from build123d import *

# Parameters (mm, degrees)
F2_SIZE       = 2.54
F3_W          = 50.8
F3_H          = 7.62
F4_DEPTH      = 42.672
F6_R          = 3.9624
F7_DEPTH      = 38.608
F7_DEPTH_BACK = 9.398
F8_COUNT      = 8


with BuildPart() as f1:
    # F0 (on Top) → F1 (revolve)
    with BuildSketch(Plane.XY):
        Polygon((0, 25.4), (0, 44.45), (-15.748, 44.45), (-15.748, 12.7), (38.1, 12.7), (38.1, 19.05), (23.241, 19.05), (23.241, 25.4), align=None)
    revolve(axis=Axis((76.2, 0, 0), (1, 0, 0)))

    # F2
    f2_edges = [f1.edges().sort_by_distance(p)[0] for p in [
        (38.1, -19.05, 0),
        (23.241, -25.4, 0),
        (-15.748, -44.45, 0),
    ]]
    chamfer(f2_edges, length=F2_SIZE)


with BuildPart() as f4:
    # F3 (on Front) → F4 (new body, symmetric)
    with BuildSketch(Plane.XZ):
        with Locations((53.34, 0)):
            Rectangle(F3_W, F3_H)
    extrude(amount=F4_DEPTH, both=True)


with BuildPart() as f1_1:
    add(f1.part)

    # F5: cut F4
    add(f4.part, mode=Mode.SUBTRACT)


with BuildPart() as f7:
    # F6 (on face) → F7 (new body, two sides)
    with BuildSketch(Plane.YZ) as f7_sk:
        with Locations((0, -38.735)):
            Circle(F6_R)
    extrude(amount=-F7_DEPTH)
    extrude(f7_sk.sketch, amount=F7_DEPTH_BACK)


with BuildPart() as f8_1:
    # F8: instance of F7
    add(f7.part.rotate(Axis((-15.748, 0, 0), (1, 0, 0)), 1 * 360 / F8_COUNT))


with BuildPart() as f8_2:
    # F8: instance of F7
    add(f7.part.rotate(Axis((-15.748, 0, 0), (1, 0, 0)), 2 * 360 / F8_COUNT))


with BuildPart() as f8_3:
    # F8: instance of F7
    add(f7.part.rotate(Axis((-15.748, 0, 0), (1, 0, 0)), 3 * 360 / F8_COUNT))


with BuildPart() as f8_4:
    # F8: instance of F7
    add(f7.part.rotate(Axis((-15.748, 0, 0), (1, 0, 0)), 4 * 360 / F8_COUNT))


with BuildPart() as f8_5:
    # F8: instance of F7
    add(f7.part.rotate(Axis((-15.748, 0, 0), (1, 0, 0)), 5 * 360 / F8_COUNT))


with BuildPart() as f8_6:
    # F8: instance of F7
    add(f7.part.rotate(Axis((-15.748, 0, 0), (1, 0, 0)), 6 * 360 / F8_COUNT))


with BuildPart() as f8_7:
    # F8: instance of F7
    add(f7.part.rotate(Axis((-15.748, 0, 0), (1, 0, 0)), 7 * 360 / F8_COUNT))


with BuildPart() as f1_2:
    add(f1_1.part)

    # F9: cut F8_5, F7, F8_1, F8_4, F8_7, F8_6, F8_2, F8_3
    add(f8_5.part, mode=Mode.SUBTRACT)
    add(f7.part, mode=Mode.SUBTRACT)
    add(f8_1.part, mode=Mode.SUBTRACT)
    add(f8_4.part, mode=Mode.SUBTRACT)
    add(f8_7.part, mode=Mode.SUBTRACT)
    add(f8_6.part, mode=Mode.SUBTRACT)
    add(f8_2.part, mode=Mode.SUBTRACT)
    add(f8_3.part, mode=Mode.SUBTRACT)


solid = f1_2.part
Work out the finished part from the listing and answer in its coordinate system (mm). A direction names the side the tool comes from. Round coordinates to 2 decimals unless told otherwise and drop trailing zeros. Write each loop counter-clockwise with the first axis right and the second up, starting at its lowest first coordinate (ties: lowest second). Pieces come first, ordered by that corner, then holes. Notation, with made-up numbers: (13.25, -39) -> (70.25, -39) arc R26 cw to (70.25, -25) -> close; hole circle Ø2 at (62.5, 18.25). An arc over 180 degrees is marked (long way). Answer as CSV lines item,"result". Start each with the question number.
(1) A tool of negligible diameter and unlimited length cuts with its end or side. For faces 4 (the cylindrical face through (29.31, 18.17, 5.72)), 5 (the flat face through (33, -15, 3.81)), 6 (the cylindrical face through (-7.8, -30.1, -24.5)), from which of +Z, -Z, +X, -X, +Y, -Y can it reach the whole face along a straight path? Write none if from no direction.
(2) Each of these flat-tipped pins is pushed along its axis until it touches: pin 1 (10.5 mm diameter, centred on y = -27.39, z = -27.39, fed in from -X); pin 2 (12 mm diameter, centred on x = 19, y = 8.5, fed in from +Z); pin 3 (10 mm diameter, centred on x = 9, z = -16.5, fed in from -Y); pin 4 (10 mm diameter, centred on x = 19, z = -26, fed in from -Y). Where does it stop, or does it pass through?
(3) The part is cut by section A-A, the plane z = 0. Give the vertices of the cut face in (x, y).
(4) The part is cut by section C-C, the plane y = 0. Give the vertices of the cut face in (x, z).
(5) Find the intervals of material crossed by probe 1 along Z at (x, y) = (-6, 0); probe 2 along Z at (x, y) = (-1.5, -1); probe 3 along Z at (x, y) = (-8.5, 26.5), in increasing order.
(6) The part is cut by section B-B, the plane x = -7.5. Give the number of separate pieces and of enclosed holes in the cut face, then the cut area to 3 significant figures.
(7) The mould has two halves that part along Y. Classify faces 1 (the cylindrical face through (-6.696, 42.397, 13.352)), 2 (the flat face through (27.94, 16, 0)), 3 (the cylindrical face through (-7.8, 24.5, -30.1)): +Y half, -Y half, draft (parallel to the pull), parting line (faces both ways), or undercut.
Output values:
1,face 4,"+X"
1,face 5,"+X, +Y, -Y"
1,face 6,"+X, -X"
2,pin 1,"stops at x = -15.75"
2,pin 2,"stops at z = 25.28"
2,pin 3,"stops at y = -22.65"
2,pin 4,"stops at y = -14.29"
3,outline,"(-15.75, -34.77) -> (0, -34.77) -> (0, -25.4) -> (20.7, -25.4) -> (23.24, -22.86) -> (23.24, -19.05) -> (27.94, -19.05) -> (27.94, -12.7) -> (-15.75, -12.7) -> close; (-15.75, 12.7) -> (27.94, 12.7) -> (27.94, 19.05) -> (23.24, 19.05) -> (23.24, 22.86) -> (20.7, 25.4) -> (0, 25.4) -> (0, 34.77) -> (-15.75, 34.77) -> close; (-14.96, -42.7) -> (-13.21, -44.45) -> (0, -44.45) -> (0, -42.7) -> close; (-14.96, 42.7) -> (0, 42.7) -> (0, 44.45) -> (-13.21, 44.45) -> close"
4,outline,"(-15.75, -34.77) -> (0, -34.77) -> (0, -25.4) -> (20.7, -25.4) -> (23.24, -22.86) -> (23.24, -19.05) -> (35.56, -19.05) -> (38.1, -16.51) -> (38.1, -12.7) -> (-15.75, -12.7) -> close; (-15.75, 12.7) -> (38.1, 12.7) -> (38.1, 16.51) -> (35.56, 19.05) -> (23.24, 19.05) -> (23.24, 22.86) -> (20.7, 25.4) -> (0, 25.4) -> (0, 34.77) -> (-15.75, 34.77) -> close; (-14.96, -42.7) -> (-13.21, -44.45) -> (0, -44.45) -> (0, -42.7) -> close; (-14.96, 42.7) -> (0, 42.7) -> (0, 44.45) -> (-13.21, 44.45) -> close"
5,probe 1,"z = -44.45 to -42.7, -34.77 to -12.7, 12.7 to 34.77, 42.7 to 44.45"
5,probe 2,"z = -44.44 to -42.57, -34.9 to -12.66, 12.66 to 34.9, 42.57 to 44.44"
5,probe 3,"z = -35.69 to -31.25, -23.53 to 23.53, 31.25 to 35.69"
6,separate pieces,"1"
6,enclosed holes,"9"
6,area,"5,310 mm²"
7,face 1,"parting line"
7,face 2,"draft"
7,face 3,"undercut"
